Input: part model. Units: mm. Frame: model coordinates. A direction names the side the tool comes from. Give positions to 0.01 mm unless a question says otherwise; leave off trailing zeros. Write each loop counter-clockwise with the first axis right and the second up, starting at its lowest first coordinate (ties: lowest second). Pieces come first, ordered by that corner, then holes. Notation, with made-up numbers: (43.25, 78) - (64.25, 78) arc R16 ccw to (64.25, 82) - close; hole circle Ø8 at (64, -6.5). An arc over 180 degrees is marked (long way). Use a Markdown table: item, result. Add a question column.
1. Material intervals for probe 1 along Y at (x, z) = (50, 15.5); probe 2 along Y at (x, z) = (44.5, 18); probe 3 along Z at (x, y) = (0, 66), sorted ascending.
2. Set-up query: faces 1 (the cylindrical face through (130.98, -1.78, -18.67)), 2 (the cylindrical face through (-8.767, 103.669, -16.856)), 3 (the flat face through (-120, -90, 4)). Return all of +Z, -Z, +X, -X, +Y, -Y with unobstructed straight access to the full face (end or side cutting, diameter ignored); none if empty.
3. Section query A-A, the plane y = 40. Return loops of the section in (x, z).
4. Mould query, pull axis X, two halves, no side actions, for faces 4 (the flat face through (135, 95, 0)), 5 (the flat face through (50, -95, 10)), 6 (the flat face through (-23, 94, -20)). Classes: released by +X, released by -X, zero draft, split by the parting line, or undercut.
5. Pin query (flat end, axial travel): pin 1 (4 mm diameter, centred on x = 121, y = -90, fed in from +Z); pin 2 (5 mm diameter, centred on x = -50, y = 95, fed in from +Z). Return the tip coordinate at first contact, or that it passes through.
6. Section query C-C, the plane x = -70. Count the separate pieces of the cut face and the enclosed holes in it, plus the area to 3 significant figures.
7. Section query B-B, the plane y = 8. Return loops of the section in (x, z), plus the area to 3 significant figures.
```python
from build123d import *

# Parameters (mm, degrees)
F0_W          = 300
F0_H          = 210
F1_DEPTH      = 20
F1_DEPTH_BACK = 20
F2_R          = 12.5
F3_DEPTH      = 105
F3_DEPTH_BACK = 105
F4_R          = 19
F4_R_2        = 14
F5_DEPTH      = 2.7
F6_R          = 19
F6_R_2        = 14
F7_DEPTH      = 2.7
F8_R          = 6.5
F8_R_2        = 4.25
F9_DEPTH      = 20
F8_R_3        = 3
F10_DEPTH     = 10
F8_R_4        = 5
F11_DEPTH     = 40
F8_R_5        = 4
F12_DEPTH     = 16
F13_SIZE      = 25
F14_R         = 1.5875
F14_R_2       = 1.5
F15_DEPTH     = 10
F16_DEPTH     = 40
F4_R_3        = 1.5875
F4_R_4        = 1.5
F17_DEPTH     = 10
F18_DEPTH     = 40
F6_R_3        = 1.5
F19_DEPTH     = 40
F20_R         = 1.5
F21_DEPTH     = 70
F22_R         = 1.5
F23_DEPTH     = 70
F4_R_5        = 2.5
F24_DEPTH     = 10
F26_DEPTH     = 2.7
F28_DEPTH     = 2.7


with BuildPart() as f1:
    # F0 (on Top) → F1 (new body, two sides)
    with BuildSketch(Plane.XY) as f1_sk:
        Rectangle(F0_W, F0_H)
        with BuildLine():
            ThreePointArc((-50, -86), (-136, 0), (-50, 86))
            Line((-50, 86), (50, 86))
            ThreePointArc((50, 86), (136, 0), (50, -86))
            Line((50, -86), (-50, -86))
        make_face(mode=Mode.SUBTRACT)
        with BuildLine():
            Line((50, 86), (-50, 86))
            ThreePointArc((-50, 86), (-136, 0), (-50, -86))
            Line((-50, -86), (50, -86))
            ThreePointArc((50, -86), (136, 0), (50, 86))
        make_face()
        with BuildLine():
            ThreePointArc((-50, -81), (-131, 0), (-50, 81))
            Line((-50, 81), (50, 81))
            ThreePointArc((50, 81), (131, 0), (50, -81))
            Line((50, -81), (-50, -81))
        make_face(mode=Mode.SUBTRACT)
        with BuildLine():
            Line((50, 81), (-50, 81))
            ThreePointArc((-50, 81), (-131, 0), (-50, -81))
            Line((-50, -81), (50, -81))
            ThreePointArc((50, -81), (131, 0), (50, 81))
        make_face()
        with BuildLine():
            ThreePointArc((0, -54.6611964743), (-124.08, 0), (0, 54.6611964743))
            ThreePointArc((0, 54.6611964743), (124.08, 0), (0, -54.6611964743))
        make_face(mode=Mode.SUBTRACT)
    extrude(amount=F1_DEPTH)
    extrude(f1_sk.sketch, amount=-F1_DEPTH_BACK)

    # F2 (on Front) → F3 (cut, two sides)
    with BuildSketch(Plane.XZ) as f3_sk:
        Circle(F2_R)
    extrude(amount=-F3_DEPTH, mode=Mode.SUBTRACT)
    extrude(f3_sk.sketch, amount=F3_DEPTH_BACK, mode=Mode.SUBTRACT)

    # F4 (on face) → F5 (cut)
    with BuildSketch(Plane.XZ.offset(105)):
        Circle(F4_R)
        Circle(F4_R_2, mode=Mode.SUBTRACT)
    extrude(amount=-F5_DEPTH, mode=Mode.SUBTRACT)

    # F6 (on face) → F7 (cut)
    with BuildSketch(Plane(origin=(0, 105, 0), x_dir=(-1, 0, 0), z_dir=(0, 1, 0))):
        Circle(F6_R)
        Circle(F6_R_2, mode=Mode.SUBTRACT)
    extrude(amount=-F7_DEPTH, mode=Mode.SUBTRACT)

    # F8 (on face) → F9 (cut)
    with BuildSketch(Plane.XY.offset(20)):
        with Locations((140, 50)):
            Circle(F8_R)
        with Locations((140, 50)):
            Circle(F8_R_2, mode=Mode.SUBTRACT)
        with Locations((140, -50)):
            Circle(F8_R)
        with Locations((140, -50)):
            Circle(F8_R_2, mode=Mode.SUBTRACT)
        with Locations((70, -95)):
            Circle(F8_R)
        with Locations((70, -95)):
            Circle(F8_R_2, mode=Mode.SUBTRACT)
        with Locations((-70, -95)):
            Circle(F8_R)
        with Locations((-70, -95)):
            Circle(F8_R_2, mode=Mode.SUBTRACT)
        with Locations((-140, -50)):
            Circle(F8_R)
        with Locations((-140, -50)):
            Circle(F8_R_2, mode=Mode.SUBTRACT)
        with Locations((-140, 50)):
            Circle(F8_R)
        with Locations((-140, 50)):
            Circle(F8_R_2, mode=Mode.SUBTRACT)
        with Locations((-70, 95)):
            Circle(F8_R)
        with Locations((-70, 95)):
            Circle(F8_R_2, mode=Mode.SUBTRACT)
        with Locations((70, 95)):
            Circle(F8_R)
        with Locations((70, 95)):
            Circle(F8_R_2, mode=Mode.SUBTRACT)
    extrude(amount=-F9_DEPTH, mode=Mode.SUBTRACT)

    # F8 (on face) → F10 (cut)
    with BuildSketch(Plane.XY.offset(20)):
        with Locations((-50, 95)):
            Circle(F8_R_3)
        with Locations((-145, 0)):
            Circle(F8_R_3)
        with Locations((50, 95)):
            Circle(F8_R_3)
        with Locations((145, 0)):
            Circle(F8_R_3)
        with Locations((-50, -95)):
            Circle(F8_R_3)
        with Locations((50, -95)):
            Circle(F8_R_3)
    extrude(amount=-F10_DEPTH, mode=Mode.SUBTRACT)

    # F8 (on face) → F11 (cut)
    with BuildSketch(Plane.XY.offset(20)):
        with Locations((-70, 95)):
            Circle(F8_R_2)
        with Locations((-140, 50)):
            Circle(F8_R_2)
        with Locations((-140, -50)):
            Circle(F8_R_2)
        with Locations((-70, -95)):
            Circle(F8_R_2)
        with Locations((70, -95)):
            Circle(F8_R_2)
        with Locations((140, -50)):
            Circle(F8_R_2)
        with Locations((140, 50)):
            Circle(F8_R_2)
        with Locations((70, 95)):
            Circle(F8_R_2)
        with Locations((-140, 70)):
            Circle(F8_R_4)
        with Locations((140, -70)):
            Circle(F8_R_4)
    extrude(amount=-F11_DEPTH, mode=Mode.SUBTRACT)

    # F8 (on face) → F12 (cut)
    with BuildSketch(Plane.XY.offset(20)):
        with Locations((-120, 90)):
            Circle(F8_R_5)
        with Locations((-120, -90)):
            Circle(F8_R_5)
        with Locations((120, -90)):
            Circle(F8_R_5)
        with Locations((120, 90)):
            Circle(F8_R_5)
    extrude(amount=-F12_DEPTH, mode=Mode.SUBTRACT)

    # F13
    f13_edges = [f1.edges().sort_by_distance(p)[0] for p in [
        (-150, 105, 0),
        (-150, -105, 0),
        (150, 105, 0),
        (150, -105, 0),
    ]]
    chamfer(f13_edges, length=F13_SIZE)

    # F14 (on face) → F15 (cut)
    with BuildSketch(Plane.YZ.offset(150)):
        Circle(F14_R)
        Circle(F14_R_2, mode=Mode.SUBTRACT)
    extrude(amount=-F15_DEPTH, mode=Mode.SUBTRACT)

    # F16 (cut): a face of the model
    f16_faces = [f1.faces().sort_by_distance(p)[0] for p in [
        (150, 0, 0),
    ]]
    extrude(f16_faces, amount=-F16_DEPTH, mode=Mode.SUBTRACT)

    # F4 (on face) → F17 (cut)
    with BuildSketch(Plane.XZ.offset(105)):
        with Locations((50, 0)):
            Circle(F4_R_3)
        with Locations((50, 0)):
            Circle(F4_R_4, mode=Mode.SUBTRACT)
    extrude(amount=-F17_DEPTH, mode=Mode.SUBTRACT)

    # F4 (on face) → F18 (cut)
    with BuildSketch(Plane.XZ.offset(105)):
        with Locations((50, 0)):
            Circle(F4_R_4)
    extrude(amount=-F18_DEPTH, mode=Mode.SUBTRACT)

    # F6 (on face) → F19 (cut)
    with BuildSketch(Plane(origin=(0, 105, 0), x_dir=(-1, 0, 0), z_dir=(0, 1, 0))):
        with Locations((-50, 0)):
            Circle(F6_R_3)
    extrude(amount=-F19_DEPTH, mode=Mode.SUBTRACT)

    # F20 (on face) → F21 (cut)
    with BuildSketch(Plane(origin=(115, -115, 0), x_dir=(0.7071067812, 0.7071067812, 0), z_dir=(0.7071067812, -0.7071067812, 0))):
        with Locations((31.8221356237, 0)):
            Circle(F20_R)
    extrude(amount=-F21_DEPTH, mode=Mode.SUBTRACT)

    # F22 (on face) → F23 (cut)
    with BuildSketch(Plane(origin=(115, 115, 0), x_dir=(-0.7071067812, 0.7071067812, 0), z_dir=(0.7071067812, 0.7071067812, 0))):
        with Locations((-31.8174746831, 0)):
            Circle(F22_R)
    extrude(amount=-F23_DEPTH, mode=Mode.SUBTRACT)

    # F4 (on face) → F24 (cut)
    with BuildSketch(Plane.XZ.offset(105)):
        with Locations((-20, 15)):
            Circle(F4_R_5)
        with Locations((20, 15)):
            Circle(F4_R_5)
        with Locations((20, -15)):
            Circle(F4_R_5)
        with Locations((-20, -15)):
            Circle(F4_R_5)
    extrude(amount=-F24_DEPTH, mode=Mode.SUBTRACT)

    # F25 (on face) → F26 (cut)
    with BuildSketch(Plane.XY.offset(20)):
        with BuildLine():
            Line((-50, -86), (50, -86))
            ThreePointArc((50, -86), (136, 0), (50, 86))
            Line((50, 86), (-50, 86))
            ThreePointArc((-50, 86), (-136, 0), (-50, -86))
        make_face()
        with BuildLine():
            ThreePointArc((50, 81), (131, 0), (50, -81))
            Line((50, -81), (-50, -81))
            ThreePointArc((-50, -81), (-131, 0), (-50, 81))
            Line((-50, 81), (50, 81))
        make_face(mode=Mode.SUBTRACT)
    extrude(amount=-F26_DEPTH, mode=Mode.SUBTRACT)

    # F27 (on face) → F28 (cut)
    with BuildSketch(Plane(origin=(0, 0, -20), x_dir=(1, 0, 0), z_dir=(0, 0, -1))):
        with BuildLine():
            Line((50, 86), (-50, 86))
            ThreePointArc((-50, 86), (-136, 0), (-50, -86))
            Line((-50, -86), (50, -86))
            ThreePointArc((50, -86), (136, 0), (50, 86))
        make_face()
        with BuildLine():
            ThreePointArc((-50, -81), (-131, 0), (-50, 81))
            Line((-50, 81), (50, 81))
            ThreePointArc((50, 81), (131, 0), (50, -81))
            Line((50, -81), (-50, -81))
        make_face(mode=Mode.SUBTRACT)
    extrude(amount=-F28_DEPTH, mode=Mode.SUBTRACT)


solid = f1.part
```
Result sheet:
| question | item | result |
|---|---|---|
| 1 | probe 1 | y = -105 to -98, -92 to -74.08, 74.08 to 92, 98 to 105 |
| 1 | probe 2 | y = -105 to -86, -81 to -73.88, 73.88 to 81, 86 to 105 |
| 1 | probe 3 | z = -20 to -12.5, 12.5 to 20 |
| 2 | face 1 | -Z |
| 2 | face 2 | +Y |
| 2 | face 3 | +Z |
| 3 | outline | (-150, -20) - (-126.13, -20) - (-126.13, -17.3) - (-120.43, -17.3) - (-120.43, -20) - (-112.35, -20) - (-112.35, 20) - (-120.43, 20) - (-120.43, 17.3) - (-126.13, 17.3) - (-126.13, 20) - (-150, 20) - close; (112.35, -20) - (120.43, -20) - (120.43, -17.3) - (126.13, -17.3) - (126.13, -20) - (150, -20) - (150, 20) - (126.13, 20) - (126.13, 17.3) - (120.43, 17.3) - (120.43, 20) - (112.35, 20) - close |
| 4 | face 4 | released by +X |
| 4 | face 5 | undercut |
| 4 | face 6 | zero draft |
| 5 | pin 1 | stops at z = 4 |
| 5 | pin 2 | stops at z = 10 |
| 6 | separate pieces | 4 |
| 6 | enclosed holes | 0 |
| 6 | area | 1,780 mm² |
| 7 | outline | (-150, -20) - (-135.63, -20) - (-135.63, -17.3) - (-130.6, -17.3) - (-130.6, -20) - (-123.65, -20) - (-123.65, 20) - (-130.6, 20) - (-130.6, 17.3) - (-135.63, 17.3) - (-135.63, 20) - (-150, 20) - close; (123.65, -20) - (130.6, -20) - (130.6, -17.3) - (135.63, -17.3) - (135.63, -20) - (150, -20) - (150, 20) - (135.63, 20) - (135.63, 17.3) - (130.6, 17.3) - (130.6, 20) - (123.65, 20) - close |
| 7 | area | 2,050 mm² |
